from build123d import *

# Parameters (mm, degrees)
CORTAR_EXTRUIR1_DEPTH = 2
CHAFL_N1_SIZE         = 0.5
REDONDEO1_R           = 0.5


with BuildPart() as part:
    # Croquis1 → Revolución1 (revolve)
    with BuildSketch(Plane.XY):
        Polygon((0, 0), (2.75, 0), (2.75, -3), (1.5, -3), (1.5, -21), (0, -21), align=None)
    revolve(axis=Axis((0, 0, 0), (0, -1, 0)))

    # Croquis2 → Cortar-Extruir1 (cut)
    with BuildSketch(Plane(origin=(0, 0, 0), x_dir=(1, 0, 0), z_dir=(0, 1, 0))):
        Polygon((1.25, 0.721687836), (0, 1.443375673), (-1.25, 0.721687836), (-1.25, -0.721687836), (0, -1.443375673), (1.25, -0.721687836), align=None)
    extrude(amount=-CORTAR_EXTRUIR1_DEPTH, mode=Mode.SUBTRACT)

    # Chaflán1
    chafl_n1_edges = [part.edges().sort_by_distance(p)[0] for p in [
        (-1.5, -21, 0),
    ]]
    chamfer(chafl_n1_edges, length=CHAFL_N1_SIZE)

    # Redondeo1
    redondeo1_edges = [part.edges().sort_by_distance(p)[0] for p in [
        (-2.75, 0, 0),
    ]]
    fillet(redondeo1_edges, radius=REDONDEO1_R)


solid = part.part
The model under review builds one solid part; all positions refer to its coordinate system, in mm. A direction names the side the tool comes from. Give positions to 0.01 mm unless a question says otherwise; leave off trailing zeros. Order: outer loops, then holes, each group sorted by start corner. A loop starts at its lowest first (then second) coordinate and runs counter-clockwise, first axis right, second up. Notation, with made-up numbers: M 31,58.5 L 42,58.5 A13 cw 42,68.5 Z; hole C -0.75,-35.75 d5. An arc over 180 degrees is marked long. Answer in a Markdown table with one row per item. Add a question column.
1. Mouldability with a two-part tool opening along Z and no side actions: class faces 4 (the cylindrical face through (-1.5, -11.87, 0.07)), 5 (the flat face through (0, -2, 0)), 6 (the flat face through (0, -21, 0)), 7 (the flat face through (1.25, -1, 0)) as released by +Z, released by -Z, zero draft, split by the parting line, or undercut.
2. Add section B-B on y = -14.5. State the section outline as (x, z) points, plus the area to 3 significant figures.
3. Machinability: for faces 1 (the flat face through (1.2, -3, -1.2)), 2 (the flat face through (-0.616, -0.986, -1.088)), 3 (the cylindrical face through (-0.596, -1.768, -2.685)), which of the approach directions +Z, -Z, +X, -X, +Y, -Y give a long, thin tool a straight path to every point of the face, cutting with its end or side? Answer none if there is none.
4. Add section A-A on z = 0. State the section outline as (x, y) points.
5. For pin 1 Ø2 at (y, z) = (-12.5, 1) entering from +X; pin 2 Ø1.5 at (x, z) = (1.5, -1) entering from -Y; pin 3 Ø3 at (x, z) = (0, 0) entering from +Y; pin 4 Ø1 at (x, y) = (-1.5, -12) entering from +Z, all flat-tipped, find the tip position at first contact; note any pin that passes through.
6. To check wall thickness, follow line 1 along Y through (x, z) = (2.15, -0.6); line 2 along X through (y, z) = (-10.25, 0.1); line 3 along Y through (x, z) = (1.4, -0.2). State the ranges of each line that lie inside material, in increasing order.
The answers:
| question | item | result |
|---|---|---|
| 1 | face 4 | split by the parting line |
| 1 | face 5 | undercut |
| 1 | face 6 | zero draft |
| 1 | face 7 | undercut |
| 2 | outline | C 0,0 d3 |
| 2 | area | 7.07 mm2 |
| 3 | face 1 | -Y |
| 3 | face 2 | +Y |
| 3 | face 3 | +Y, -Y |
| 4 | outline | M -2.75,-3 L -1.5,-3 L -1.5,-20.5 L -1,-21 L 1,-21 L 1.5,-20.5 L 1.5,-3 L 2.75,-3 L 2.75,-0.5 A0.5 ccw 2.25,0 L 1.25,0 L 1.25,-2 L -1.25,-2 L -1.25,0 L -2.25,0 A0.5 ccw -2.75,-0.5 Z |
| 5 | pin 1 | x = 1.5 |
| 5 | pin 2 | y = -20.95 |
| 5 | pin 3 | y = 0 |
| 5 | pin 4 | z = 1.12 |
| 6 | line 1 | -3 to 0 |
| 6 | line 2 | -1.5 to 1.5 |
| 6 | line 3 | -20.59 to 0 |
